Work out the finished part from the listing and answer in its coordinate system (mm). Face numbers are marked on the shaded views. A direction names the side the tool comes from. Give positions to 0.01 mm unless a question says otherwise; leave off trailing zeros. Loops run counter-clockwise (first coordinate to the right, second up) from the corner with the lowest first, then second, coordinate; pieces in that order, holes last. Notation, with made-up numbers: (24, 8.5) - (63, 8.5) arc R11 cw to (63, 20.5) - close; hole circle Ø4 at (32.25, 67.5). An arc over 180 degrees is marked (long way). Use CSV: the item, a comma, the result in double quotes.
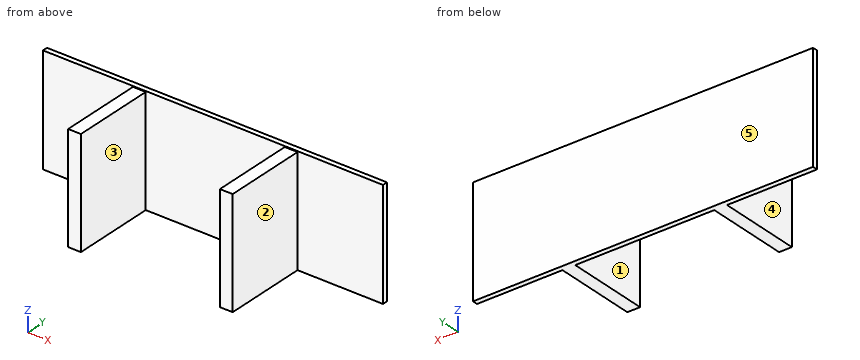
from build123d import *

# Parameters (mm, degrees)
F0_W     = 8.9696688134
F0_H     = 6
F0_W_2   = 6.0303311866
F0_W_3   = 7.6489803101
F0_W_4   = 7.3510196899
F2_DEPTH = 128
F4_DEPTH = 127


# Not quite as in the source:
# - the program builds the solid bodies; features that only make, move or delete a surface that nothing else refers to are left out


with BuildPart() as f2:
    # F0 (on Top) → F2 (new body)
    with BuildSketch(Plane.XY):
        Polygon((-400, 0), (-294.1345971149, 0), (-294.1345971149, 6), (-299.6463162062, 6), (-311.9468285562, 6), (-322.7511938045, 6), (-335.9566328529, 6), (-348.7171674377, 6), (-362.4063217106, 6), (-376.9397732412, 6), (-400, 6), align=None)
        with Locations((-283.6194315216, 3)):
            Rectangle(F0_W, F0_H)
        with Locations((-291.1194315216, 3)):
            Rectangle(F0_W_2, F0_H)
        Polygon((-279.1345971149, 0), (-115.5724730993, 0), (-115.5724730993, 6), (-120.0142995768, 6), (-130.6865749399, 6), (-142.439753188, 6), (-152.7159749868, 6), (-164.8405666594, 6), (-175.9109262937, 6), (-188.4297876225, 6), (-205.2331021726, 6), (-216.1265840576, 6), (-227.5328489064, 6), (-240.1054796123, 6), (-251.4180912129, 6), (-260.7190593146, 6), (-272.6732546984, 6), (-279.1345971149, 6), align=None)
        with Locations((-111.7479829443, 3)):
            Rectangle(F0_W_3, F0_H)
        with Locations((-104.2479829443, 3)):
            Rectangle(F0_W_4, F0_H)
        Polygon((-100.5724730993, 0), (0, 0), (0, 6), (-21.7185619105, 6), (-32.3376952831, 6), (-47.4983571934, 6), (-60.9528624883, 6), (-73.3657559167, 6), (-83.3882540464, 6), (-97.7746488723, 6), (-100.5724730993, 6), align=None)
    extrude(amount=F2_DEPTH)

    # F0 (on Top) → F4 (join)
    with BuildSketch(Plane.XY):
        Polygon((-279.1345971149, -97.6634095667), (-279.1345971149, 0), (-288.1042659283, 0), (-294.1345971149, 0), (-294.1345971149, -97.6634095667), align=None)
        Polygon((-100.5724730993, -97.6634095667), (-100.5724730993, 0), (-107.9234927893, 0), (-115.5724730993, 0), (-115.5724730993, -97.6634095667), align=None)
    extrude(amount=F4_DEPTH)


solid = f2.part
Item 1: A cutting plane is placed at B-B on z = 64.5. Determine the outline of the cut face in (x, y).
Determined:
outline,"(-400, 0) - (-294.13, 0) - (-294.13, -97.66) - (-279.13, -97.66) - (-279.13, 0) - (-115.57, 0) - (-115.57, -97.66) - (-100.57, -97.66) - (-100.57, 0) - (0, 0) - (0, 6) - (-400, 6) - close"
Item 2: A cutting plane is placed at C-C on x = -56. Determine the outline of the cut face in (y, z).
Determined:
outline,"(0, 0) - (6, 0) - (6, 128) - (0, 128) - close"
Item 3: The mould has two halves that part along X. Classify the marked faces 3, 4 and 5: pulls with the +X half, pulls with the -X half, needs draft (parallel to the pull), parting line crosses it, or undercut.
Determined:
face 3,"undercut"
face 4,"pulls with the -X half"
face 5,"needs draft"
Item 4: For the marked faces 1 and 2, determine the directions among +Z, -Z, +X, -X, +Y, -Y from which every point of the face is accessible in a straight line to the end or side of a thin tool.
Determined:
face 1,"+Z, -Z, -Y"
face 2,"+Z, -Z, +X, -Y"
Item 5: Given P1, Ø4.5, axis at x = -110, y = -62, coming from the +Z side; P2, Ø10, axis at y = -76, z = 100, coming from the -X side, each flat-ended and moving along its own axis, determine where each tip first touches the part or whether it passes through.
Determined:
P1,"stops at z = 127"
P2,"stops at x = -294.13"
Item 6: Find the intervals of material crossed by line 1 (X direction, y = -80, z = 14.5); line 2 (Y direction, x = -380, z = 16), in increasing order.
Determined:
line 1,"x = -294.13 to -279.13, -115.57 to -100.57"
line 2,"y = 0 to 6"
Item 7: A cutting plane is placed at A-A on y = -37. Determine the outline of the cut face in (x, z).
Determined:
outline,"(-294.13, 0) - (-279.13, 0) - (-279.13, 127) - (-294.13, 127) - close; (-115.57, 0) - (-100.57, 0) - (-100.57, 127) - (-115.57, 127) - close"
